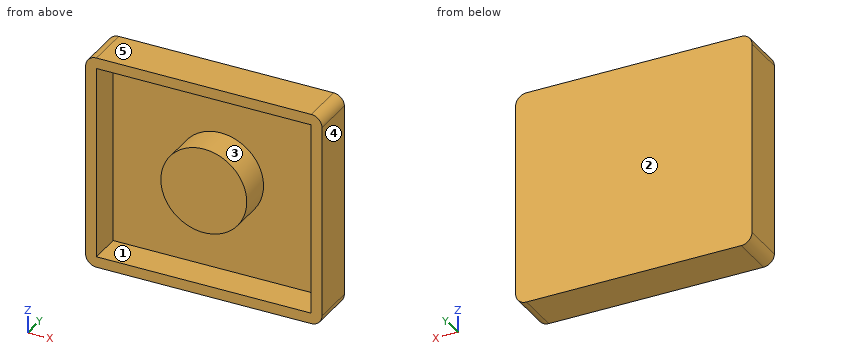
```python
from build123d import *

# Parameters (mm, degrees)
SKETCH1_W           = 13.97
SKETCH1_H           = 12.7
BOSS_EXTRUDE1_DEPTH = 2.54
FILLET1_R           = 0.635
SHELL1_START        = 0.635
SHELL1_OUTLINE_W    = 1.905
SHELL1_OUTLINE_H    = 11.43
SHELL1_DEPTH        = 12.7
SKETCH2_R           = 2.54
BOSS_EXTRUDE2_DEPTH = 1.905


# Read off the part's stored shape, not the designer's step: Shell1
with BuildPart() as part:
    # Sketch1 → Boss-Extrude1 (new body)
    with BuildSketch(Plane(origin=(0, 0, 0), x_dir=(1, 0, 0), z_dir=(0, 1, 0))):
        with Locations((6.985, 6.35)):
            Rectangle(SKETCH1_W, SKETCH1_H)
    extrude(amount=BOSS_EXTRUDE1_DEPTH)

    # Fillet1
    fillet1_edges = [part.edges().sort_by_distance(p)[0] for p in [
        (0, 1.27, -12.7),
        (13.97, 1.27, -12.7),
        (13.97, 1.27, 0),
        (0, 1.27, 0),
    ]]
    fillet(fillet1_edges, radius=FILLET1_R)

    # Shell1 outline → Shell1 (cut)
    with BuildSketch(Plane.YZ.offset(SHELL1_START)):
        with Locations((0.9525, -6.35)):
            Rectangle(SHELL1_OUTLINE_W, SHELL1_OUTLINE_H)
    extrude(amount=SHELL1_DEPTH, mode=Mode.SUBTRACT)

    # Sketch2 → Boss-Extrude2 (add)
    with BuildSketch(Plane(origin=(0, 1.905, 0), x_dir=(-1, 0, 0), z_dir=(0, -1, 0))):
        with Locations(Location((-6.985, 6.35, 0), (0, 0, 270))):
            Circle(SKETCH2_R)
    extrude(amount=BOSS_EXTRUDE2_DEPTH)


solid = part.part
```
CAD build for the part. Positions are in the model's coordinates, mm. Face numbers are marked on the shaded views. A direction names the side the tool comes from. Give positions to 0.01 mm unless a question says otherwise; leave off trailing zeros. Order: outer loops, then holes, each group sorted by start corner. A loop starts at its lowest first (then second) coordinate and runs counter-clockwise, first axis right, second up.
(1) Saw through at B-B, the plane x = 2.75. Give the cut face in (y, z) (3 decimals), then the cut area to 3 significant figures.
(2) Mould opens along Z. For the marked faces 3, 4 and 5 say: released by +Z, released by -Z, zero draft, split by the parting line, or undercut.
(3) Saw through at D-D, the plane x = 6.75. Give the cut face in (y, z) (3 decimals), then the cut area to 3 significant figures.
(4) Tool access for the marked faces 1 and 2: list every direction of +Z, -Z, +X, -X, +Y, -Y with a clear straight run to the whole face (end or side of a thin tool).
(5) Saw through at A-A, the plane y = 0.2. Give the cut face in (x, z) (3 decimals), then the cut area to 3 significant figures.
(6) Saw through at C-C, the plane z = -10.5. Give the cut face in (x, y) (3 decimals).
(7) Drill centre lines: L1, parallel to Z at x = 2.25, y = 1.4 (3 decimals); L2, parallel to X at y = 1.4, z = -10.5 (3 decimals); L3, parallel to Z at x = 6.75, y = 1.1 (3 decimals). Where is each one in solid material? Low to high.
Results found:
1. outline: (0, -12.7) - (2.54, -12.7) - (2.54, 0) - (0, 0) - (0, -0.635) - (1.905, -0.635) - (1.905, -12.065) - (0, -12.065) - close
1. area: 10.5 mm2
2. face 3: undercut
2. face 4: zero draft
2. face 5: released by +Z
3. outline: (0, -12.7) - (2.54, -12.7) - (2.54, 0) - (0, 0) - (0, -0.635) - (1.905, -0.635) - (1.905, -3.821) - (0, -3.821) - (0, -8.879) - (1.905, -8.879) - (1.905, -12.065) - (0, -12.065) - close
3. area: 20.1 mm2
4. face 1: -Y
4. face 2: +Z, -Z, +X, -X, +Y
5. outline: (0, -12.065) arc R0.635 ccw to (0.635, -12.7) - (13.335, -12.7) arc R0.635 ccw to (13.97, -12.065) - (13.97, -0.635) arc R0.635 ccw to (13.335, 0) - (0.635, 0) arc R0.635 ccw to (0, -0.635) - close; circle Ø5.08 at (6.985, -6.35); hole (0.635, -12.065) - (13.335, -12.065) - (13.335, -0.635) - (0.635, -0.635) - close
5. area: 52.2 mm2
6. outline: (0, 0) - (0.635, 0) - (0.635, 1.905) - (13.335, 1.905) - (13.335, 0) - (13.97, 0) - (13.97, 2.54) - (0, 2.54) - close
7. L1: z = -12.7 to -12.065, -0.635 to 0
7. L2: x = 0 to 0.635, 13.335 to 13.97
7. L3: z = -12.7 to -12.065, -8.879 to -3.821, -0.635 to 0
